Autodesk Inventor part; units mm, degrees
ref_plane "YZ Plane" through (0, 0, 0) normal (1, 0, 0) x (0, 1, 0)
ref_plane "XZ Plane" through (0, 0, 0) normal (0, 1, 0) x (-1, 0, 0)
ref_plane "XY Plane" through (0, 0, 0) normal (0, 0, 1) x (1, 0, 0)
sketch "Sketch1" plane through (0, 0, 0) normal (0, 0, 1) x (1, 0, 0)
  circle A0 centre (0, 0) radius 1.7526
  dimension "d0" = 3.5052
extrude "Extrusion1" add sketch "Sketch1" along normal blind 38.1
sketch "Sketch2" plane through (0, 0, 0) normal (0, 0, -1) x (-1, 0, 0)
  circle A0 centre (0, 0) radius 1.7526 construction
  circle A1 centre (0, 0) radius 2.8702
  dimension "d3" = 5.7404
extrude "Extrusion2" add sketch "Sketch2" along normal blind 3.5052
sketch "Sketch3" plane through (0, 0, -3.5052) normal (0, 0, -1) x (-1, 0, 0)
  circle A0 centre (0, 0) radius 2.8702
  line L0 (0, 1.604) -> (1.3891, 0.802)
  line L1 (1.3891, 0.802) -> (1.3891, -0.802)
  line L2 (1.3891, -0.802) -> (0, -1.604)
  line L3 (0, -1.604) -> (-1.3891, -0.802)
  line L4 (-1.3891, -0.802) -> (-1.3891, 0.802)
  line L5 (-1.3891, 0.802) -> (0, 1.604)
  dimension "d6" = 2.7781
extrude "Extrusion3" cut sketch "Sketch3" against normal blind 1.7526 contours L0 L1 L2 L3 L4 L5
chamfer "Chamfer1" distance 0.508 angle 45 1 edges at (-1.7526, 0, 38.1)
thread "Thread2"
properties part number "6-32 SHCS x1500" material "Stainless Steel"
For this review, take the finished solid that the model builds, in its own axes (mm). A direction names the side the tool comes from. Coordinates: 2 decimals unless noted, no trailing zeros. Write each loop counter-clockwise with the first axis right and the second up, starting at its lowest first coordinate (ties: lowest second). Pieces come first, ordered by that corner, then holes. Notation, with made-up numbers: (-7.5, 26.5) - (38.5, 26.5) arc R30 cw to (38.5, 51.5) - close; hole circle Ø2 at (55.25, 78.5). An arc over 180 degrees is marked (long way). Answer in a Markdown table with one row per item. Add a question column.
Q1. For probe 1 along Z at (x, y) = (-0.3, 0.05); probe 2 along X at (y, z) = (0.2, -0.5); probe 3 along Z at (x, y) = (2.2, -0.3), list the stretches that pass through material, from the lowest coordinate up.
Q2. For P1, Ø3, axis at x = -1, y = -0.5, coming from the -Z side; P2, Ø1.5, axis at x = -0.5, z = 33, coming from the -Y side, all flat-tipped, find the tip position at first contact; note any pin that passes through.
Q3. We need section A-A, the plane y = 0. State the section outline as (x, z) points, and give its area (3 significant figures).
Q4. Tool access review of faces 5 (the flat face through (-1.2, -1.2, -3.505)), 6 (the flat face through (0.7, 1.2, -2.6)), 7 (the flat face through (0, -2, 0)): name each direction out of +Z, -Z, +X, -X, +Y, -Y from which nothing blocks a thin tool from reaching the whole face with its end or side.
Q5. We need section B-B, the plane z = 34. State the section outline as (x, y) points, and give its area (3 significant figures).
Q6. Draft analysis for pull direction Y (two halves, no side actions). For faces 1 (the flat face through (0, 0, 38.1)), 2 (the flat face through (0, 0, -1.753)), 3 (the cylindrical face through (2.278, 1.746, -1.728)), 4 (the flat face through (-1.389, 0, -3)), state which applies: +Y half, -Y half, draft (parallel to the pull), parting line (faces both ways), or undercut.
Answer list:
| question | item | result |
|---|---|---|
| 1 | probe 1 | z = -1.75 to 38.1 |
| 1 | probe 2 | x = -2.86 to 2.86 |
| 1 | probe 3 | z = -3.51 to 0 |
| 2 | P1 | stops at z = -3.51 |
| 2 | P2 | stops at y = -1.75 |
| 3 | outline | (-2.87, -3.51) - (-1.39, -3.51) - (-1.39, -1.75) - (1.39, -1.75) - (1.39, -3.51) - (2.87, -3.51) - (2.87, 0) - (1.75, 0) - (1.75, 37.59) - (1.24, 38.1) - (-1.24, 38.1) - (-1.75, 37.59) - (-1.75, 0) - (-2.87, 0) - close |
| 3 | area | 149 mm2 |
| 4 | face 5 | -Z, +X, -X, +Y, -Y |
| 4 | face 6 | -Z |
| 4 | face 7 | +Z |
| 5 | outline | circle Ø3.51 at (0, 0) |
| 5 | area | 9.65 mm2 |
| 6 | face 1 | draft |
| 6 | face 2 | undercut |
| 6 | face 3 | parting line |
| 6 | face 4 | undercut |
